Geometry check sheet. Reference: the model listing, model coordinates, mm. A direction names the side the tool comes from. Give positions to 0.01 mm unless a question says otherwise; leave off trailing zeros. Loops run counter-clockwise (first coordinate to the right, second up) from the corner with the lowest first, then second, coordinate; pieces in that order, holes last. Notation, with made-up numbers: (-2.5, 45.25) -> (48.5, 45.25) arc R11 ccw to (48.5, 65.25) -> close; hole circle Ø9 at (52, 38.25). An arc over 180 degrees is marked (long way). One line per item, written item: value. Start each with the question number.
(1) Sectioned sample at D-D, the plane x = 0. Record the cut outline in (y, z), then the cut area to 3 significant figures.
(2) Sectioned sample at B-B, the plane x = -51. Record the cut outline in (y, z).
(3) Scan lines: line 1 along X through (y, z) = (-76, 9.75); line 2 along Y through (x, z) = (-50, 4.25); line 3 along Y through (x, z) = (-51, 13). Record each from-to range of solid material in increasing order. Write a range as from..to.
(4) Draft check along Y on faces 4 (the face through (-1.041, 65.932, 4.93)), 5 (the face through (-0.605, 27.493, 9.86)), 6 (the face through (19, 23, 0)). Enter one of: pulls with the +Y half, pulls with the -Y half, needs draft (parallel to the pull), parting line crosses it, or undercut.
(5) Sectioned sample at A-A, the plane z = 4.75. Record the cut outline in (x, y).
(6) Sectioned sample at C-C, the plane y = -45.5. Record the cut outline in (x, z), then the cut area to 3 significant figures.
(7) Gauge pin test, flat ends, axial feed: pin 1 Ø10 at (x, z) = (6, 5.5) entering from -Y; pin 2 Ø12 at (x, z) = (-25.5, 12) entering from +Y; pin 3 Ø5 at (x, z) = (55, 13) entering from +Y. Record the tip position at first contact, or that the pin passes through.
(8) Tool access check on faces 1 (the face through (-27.5, -43, 10)), 2 (the face through (5.2, 56.3, 10)), 3 (the face through (-55.17, -31.19, 14.93)). Record the directions out of +Z, -Z, +X, -X, +Y, -Y that give a thin tool (end or side, any length) a straight path to the whole face; none if there is none.
from build123d import *

# Parameters (mm, degrees)
F0_R     = 8
F0_R_2   = 5.25
F1_DEPTH = 20
F2_DEPTH = 20.001
F3_DEPTH = 10


with BuildPart() as f1:
    # F0 (on Top) → F1 (new body)
    with BuildSketch(Plane.XY):
        with BuildLine():
            ThreePointArc((27.5, -85.695683), (72.715198, -53.033009), (90, 0))
            ThreePointArc((90, 0), (-53.033009, 72.715198), (-27.5, -85.695683))
            Line((-27.5, -85.695683), (-27.5, 0))
            ThreePointArc((-27.5, 0), (0, 27.5), (27.5, 0))
            Line((27.5, 0), (27.5, -85.695683))
        make_face()
        with Locations((-51, -28)):
            Circle(F0_R, mode=Mode.SUBTRACT)
        with Locations((51, -28)):
            Circle(F0_R, mode=Mode.SUBTRACT)
        with Locations((0, 58)):
            Circle(F0_R, mode=Mode.SUBTRACT)
        with Locations((-51, -28)):
            Circle(F0_R_2)
        with Locations((-51, -28)):
            Circle(F0_R)
        with Locations((-51, -28)):
            Circle(F0_R_2, mode=Mode.SUBTRACT)
        with Locations((51, -28)):
            Circle(F0_R)
        with Locations((51, -28)):
            Circle(F0_R_2, mode=Mode.SUBTRACT)
        with Locations((51, -28)):
            Circle(F0_R_2)
        with Locations((0, 58)):
            Circle(F0_R)
        with Locations((0, 58)):
            Circle(F0_R_2, mode=Mode.SUBTRACT)
        with Locations((0, 58)):
            Circle(F0_R_2)
    extrude(amount=F1_DEPTH)

    # F0 (on Top) → F2 (cut, through all)
    with BuildSketch(Plane.XY):
        with Locations((0, 58)):
            Circle(F0_R_2)
        with Locations((-51, -28)):
            Circle(F0_R_2)
        with Locations((51, -28)):
            Circle(F0_R_2)
    extrude(amount=F2_DEPTH, mode=Mode.SUBTRACT)

    # F0 (on Top) → F3 (cut)
    with BuildSketch(Plane.XY):
        with Locations((0, 58)):
            Circle(F0_R)
        with Locations((0, 58)):
            Circle(F0_R_2, mode=Mode.SUBTRACT)
        with Locations((51, -28)):
            Circle(F0_R)
        with Locations((51, -28)):
            Circle(F0_R_2, mode=Mode.SUBTRACT)
        with Locations((-51, -28)):
            Circle(F0_R)
        with Locations((-51, -28)):
            Circle(F0_R_2, mode=Mode.SUBTRACT)
    extrude(amount=F3_DEPTH, mode=Mode.SUBTRACT)


solid = f1.part
Calculated:
1. outline: (27.5, 0) -> (50, 0) -> (50, 10) -> (52.75, 10) -> (52.75, 20) -> (27.5, 20) -> close; (63.25, 10) -> (66, 10) -> (66, 0) -> (90, 0) -> (90, 20) -> (63.25, 20) -> close
1. area: 985 mm2
2. outline: (-74.16, 0) -> (-36, 0) -> (-36, 10) -> (-33.25, 10) -> (-33.25, 20) -> (-74.16, 20) -> close; (-22.75, 10) -> (-20, 10) -> (-20, 0) -> (74.16, 0) -> (74.16, 20) -> (-22.75, 20) -> close
3. line 1: x = -48.21..-27.5, 27.5..48.21
3. line 2: y = -74.83..-35.94, -20.06..74.83
3. line 3: y = -74.16..-33.25, -22.75..74.16
4. face 4: undercut
4. face 5: pulls with the -Y half
4. face 6: needs draft
5. outline: (-27.5, -85.7) -> (-27.5, 0) arc R27.5 cw to (27.5, 0) -> (27.5, -85.7) arc R90 ccw (long way) to start; hole circle Ø16 at (-51, -28); hole circle Ø16 at (0, 58); hole circle Ø16 at (51, -28)
6. outline: (-77.65, 0) -> (-27.5, 0) -> (-27.5, 20) -> (-77.65, 20) -> close; (27.5, 0) -> (77.65, 0) -> (77.65, 20) -> (27.5, 20) -> close
6. area: 2,010 mm2
7. pin 1: stops at y = 25.2
7. pin 2: stops at y = 87.86
7. pin 3: stops at y = 73.1
8. face 1: +Z, -Z, -Y
8. face 2: -Z
8. face 3: +Z, -Z
